Input: part model. Units: mm. Frame: model coordinates. A direction names the side the tool comes from. Round coordinates to 2 decimals unless told otherwise and drop trailing zeros. Loops run counter-clockwise (first coordinate to the right, second up) from the corner with the lowest first, then second, coordinate; pieces in that order, holes last. Notation, with made-up numbers: (38, -19) -> (74, -19) arc R23 ccw to (74, -11) -> close; hole circle Ø9 at (-12.5, -17.75). An arc over 180 degrees is marked (long way). Answer in a Markdown table with one row per item. Add a question column.
Q1. Section D-D, the plane x = 8.75. Output: boundary loops of the cut face in (y, z).
Q2. Section B-B, the plane y = 0. Output: boundary loops of the cut face in (x, z).
Q3. Pin query (flat end, axial travel): pin 1 (1 mm diameter, centred on x = 0, y = 1, fed in from +Z); pin 2 (2 mm diameter, centred on x = 2.5, z = -26.5, fed in from +Y); pin 3 (3 mm diameter, centred on x = -1, z = -74, fed in from -Y); pin 4 (1 mm diameter, centred on x = 8, z = -66, fed in from +Y). Return the tip coordinate at first contact, or that it passes through.
Q4. Ray query, L1, parallel to Z at x = -2.5, y = -4.25; L2, parallel to Y at x = 8.75, z = -45.5; L3, parallel to X at y = -4, z = -42. Return the intervals inside material, ascending. Write a range as from..to.
Q5. Section C-C, the plane z = -64. Output: boundary loops of the cut face in (x, y), and give its area (3 significant figures).
Q6. Section A-A, the plane x = 0. Output: boundary loops of the cut face in (y, z).
Q7. Mould query, pull axis X, two halves, no side actions, for faces 4 (the face through (0, -2, 0)), 5 (the face through (10, 3.2, -57.2)), 6 (the face through (0, -1.567, -5)). Classes: pulls with the +X half, pulls with the -X half, needs draft (parallel to the pull), parting line crosses it, or undercut.
Q8. Reachability of faces 1 (the face through (0, 0, -131)), 2 (the face through (2.6, 0.1, -4.9)), 3 (the face through (5, 0, -116)) from +Z, -Z, +X, -X, +Y, -Y: full face, straight path, thin tool, end or side. Return the list, or none.
```python
from build123d import *

# Parameters (mm, degrees)
SKETCH2_R           = 10.5
BOSS_EXTRUDE1_DEPTH = 116
SKETCH3_R           = 4.45
BOSS_EXTRUDE2_DEPTH = 15
CUT_EXTRUDE1_DEPTH  = 10


with BuildPart() as part:
    # Sketch2 → Boss-Extrude1 (new body)
    with BuildSketch(Plane.XY):
        Circle(SKETCH2_R)
    extrude(amount=-BOSS_EXTRUDE1_DEPTH)

    # Sketch3 → Boss-Extrude2 (add)
    with BuildSketch(Plane(origin=(0, 0, -116), x_dir=(-1, 0, 0), z_dir=(0, 0, -1))):
        Circle(SKETCH3_R)
    extrude(amount=BOSS_EXTRUDE2_DEPTH)

    # Sketch1 → Cut-Extrude1 (cut)
    with BuildSketch(Plane.XY):
        with BuildLine():
            Line((2.051104302, -1.567413373), (-2.047676004, -1.567413373))
            ThreePointArc((-2.047676004, -1.567413373), (-2.598285851, 0.032586627), (-2.047676004, 1.632586627))
            Line((-2.047676004, 1.632586627), (2.051104302, 1.632586627))
            ThreePointArc((2.051104302, 1.632586627), (2.601714149, 0.032586627), (2.051104302, -1.567413373))
        make_face()
    extrude(amount=-CUT_EXTRUDE1_DEPTH, mode=Mode.SUBTRACT)


solid = part.part
```
Answer block:
| question | item | result |
|---|---|---|
| 1 | outline | (-5.8, -116) -> (5.8, -116) -> (5.8, 0) -> (-5.8, 0) -> close |
| 2 | outline | (-10.5, -116) -> (-4.45, -116) -> (-4.45, -131) -> (4.45, -131) -> (4.45, -116) -> (10.5, -116) -> (10.5, 0) -> (2.6, 0) -> (2.6, -10) -> (-2.6, -10) -> (-2.6, 0) -> (-10.5, 0) -> close |
| 3 | pin 1 | z = -10 |
| 3 | pin 2 | y = 10.39 |
| 3 | pin 3 | y = -10.5 |
| 3 | pin 4 | y = 7.35 |
| 4 | L1 | -116..0 |
| 4 | L2 | -5.8..5.8 |
| 4 | L3 | -9.71..9.71 |
| 5 | outline | circle Ø21 at (0, 0) |
| 5 | area | 346 mm^2 |
| 6 | outline | (-10.5, -116) -> (-4.45, -116) -> (-4.45, -131) -> (4.45, -131) -> (4.45, -116) -> (10.5, -116) -> (10.5, 0) -> (1.63, 0) -> (1.63, -10) -> (-1.57, -10) -> (-1.57, 0) -> (-10.5, 0) -> close |
| 7 | face 4 | needs draft |
| 7 | face 5 | parting line crosses it |
| 7 | face 6 | undercut |
| 8 | face 1 | -Z, +X, -X, +Y, -Y |
| 8 | face 2 | +Z |
| 8 | face 3 | -Z |
